from build123d import *

# Parameters (mm, degrees)
F0_R     = 2.5
F1_DEPTH = 7.5
F2_W     = 3.4
F2_H     = 15.4505071864
F2_W_2   = 3.8797123611
F2_W_3   = 3.8316924378
F3_DEPTH = 16.41578
F5_DEPTH = 2.8
F7_DEPTH = 2.8


with BuildPart() as f1:
    # F0 (on Right) → F1 (new body, symmetric)
    with BuildSketch(Plane.YZ):
        with BuildLine():
            Line((7.5, -12.5), (7.5, 0))
            ThreePointArc((7.5, 0), (0, 7.5), (-7.5, 0))
            Line((-7.5, 0), (-7.5, -12.5))
            Line((-7.5, -12.5), (7.5, -12.5))
        make_face()
        Circle(F0_R, mode=Mode.SUBTRACT)
    extrude(amount=F1_DEPTH, both=True)

    # F2 (on Front) → F3 (cut, symmetric)
    with BuildSketch(Plane.XZ):
        with Locations((0, 0.7252535932)):
            Rectangle(F2_W, F2_H)
        with Locations((-6.6398561805, 0.7252535932)):
            Rectangle(F2_W_2, F2_H)
        with Locations((6.6158462189, 0.7252535932)):
            Rectangle(F2_W_3, F2_H)
    extrude(amount=F3_DEPTH, both=True, mode=Mode.SUBTRACT)

    # F4 (on face) → F5 (cut, through all)
    with BuildSketch(Plane(origin=(-7.5, 0, 0), x_dir=(0, -1, 0), z_dir=(-1, 0, 0))):
        with BuildLine():
            ThreePointArc((2.6925824036, -7), (6.1824092402, -4.2459175671), (7.5, 0))
            ThreePointArc((7.5, 0), (-4.2459175671, 6.1824092402), (-2.6925824036, -7))
            Line((-2.6925824036, -7), (2.6925824036, -7))
        make_face()
        with BuildLine():
            Line((2.6925824036, -7), (-2.6925824036, -7))
            ThreePointArc((-2.6925824036, -7), (0, -7.5), (2.6925824036, -7))
        make_face()
    extrude(amount=-F5_DEPTH, mode=Mode.SUBTRACT)

    # F6 (on face) → F7 (cut, through all)
    with BuildSketch(Plane.YZ.offset(7.5)):
        with BuildLine():
            Line((2.6925824036, -7), (-2.6925824036, -7))
            ThreePointArc((-2.6925824036, -7), (0, -7.5), (2.6925824036, -7))
        make_face()
        with BuildLine():
            ThreePointArc((2.6925824036, -7), (6.1824092402, -4.2459175671), (7.5, 0))
            ThreePointArc((7.5, 0), (-4.2459175671, 6.1824092402), (-2.6925824036, -7))
            Line((-2.6925824036, -7), (2.6925824036, -7))
        make_face()
    extrude(amount=-F7_DEPTH, mode=Mode.SUBTRACT)


solid = f1.part
Verification items for the finished model (mm, model axes). A direction names the side the tool comes from. Give positions to 0.01 mm unless a question says otherwise; leave off trailing zeros. Loops run counter-clockwise (first coordinate to the right, second up) from the corner with the lowest first, then second, coordinate; pieces in that order, holes last.
1) Sectioned sample at A-A, the plane y = 0. Enter the section's corners in (x, z).
2) Sectioned sample at C-C, the plane x = 3. Enter the section's corners in (y, z), then the cut area to 3 significant figures.
3) Sectioned sample at D-D, the plane y = -6. Enter the section's corners in (x, z), then the cut area to 4 significant figures.
4) Draft check along Y on faces 6 (the flat face through (-6, 5, -7)), 7 (the cylindrical face through (3.18, -0.54, -2.44)), 8 (the cylindrical face through (3.22, 0.16, 7.5)), 9 (the cylindrical face through (-6.1, 0, -7.5)). Enter one of: pulls with the +Y half, pulls with the -Y half, needs draft (parallel to the pull), parting line crosses it, or undercut.
5) Thickness scan on line 1 along X through (y, z) = (4.25, -5.75); line 2 along Z through (x, y) = (3.8, 0); line 3 along Z through (x, y) = (-1.5, 4.5). Record the ranges inside material, lowest first.
6) Depth check by flat-ended pin: pin 1 Ø6.5 at (y, z) = (0, 0) entering from -X; pin 2 Ø0.8 at (x, y) = (-6.5, 5) entering from +Z; pin 3 Ø4.5 at (y, z) = (-1, -2) entering from +X. Enter the tip coordinate at first touch or a pass-through.
7) Set-up check for faces 1 (the flat face through (6, 5, -7)), 2 (the flat face through (0, 0, -7)), 3 (the flat face through (-6, -5, -7)), 4 (the cylindrical face through (-3.22, -0.54, -2.44)), 5 (the cylindrical face through (-3.18, 0.16, 7.5)): record each of +Z, -Z, +X, -X, +Y, -Y from which the full face is reachable in a straight line by a thin tool's end or side.
8) Sectioned sample at B-B, the plane z = -6.5. Enter the section's corners in (x, y), then the cut area to 3 significant figures.
Answers:
1. outline: (-7.5, -12.5) - (7.5, -12.5) - (7.5, -7.5) - (4.7, -7.5) - (4.7, -2.5) - (1.7, -2.5) - (1.7, -7) - (-1.7, -7) - (-1.7, -2.5) - (-4.7, -2.5) - (-4.7, -7.5) - (-7.5, -7.5) - close; (-4.7, 2.5) - (-1.7, 2.5) - (-1.7, 7.5) - (-4.7, 7.5) - close; (1.7, 2.5) - (4.7, 2.5) - (4.7, 7.5) - (1.7, 7.5) - close
2. outline: (-7.5, -12.5) - (7.5, -12.5) - (7.5, 0) arc R7.5 ccw to (-7.5, 0) - close; hole circle Ø5 at (0, 0)
2. area: 256 mm2
3. outline: (-7.5, -12.5) - (7.5, -12.5) - (7.5, -7) - (4.7, -7) - (4.7, 4.5) - (1.7, 4.5) - (1.7, -7) - (-1.7, -7) - (-1.7, 4.5) - (-4.7, 4.5) - (-4.7, -7) - (-7.5, -7) - close
3. area: 151.5 mm2
4. face 6: needs draft
4. face 7: undercut
4. face 8: parting line crosses it
4. face 9: undercut
5. line 1: x = -4.7 to -1.7, 1.7 to 4.7
5. line 2: z = -12.5 to -2.5, 2.5 to 7.5
5. line 3: z = -12.5 to -7
6. pin 1: stops at x = -4.7
6. pin 2: stops at z = -7
6. pin 3: stops at x = 4.7
7. face 1: +Z, +X, +Y, -Y
7. face 2: +Z, +Y, -Y
7. face 3: +Z, -X, +Y, -Y
7. face 4: +X, -X
7. face 5: +Z, +X, -X
8. outline: (-4.7, -7.5) - (-1.7, -7.5) - (-1.7, 7.5) - (-4.7, 7.5) - close; (1.7, -7.5) - (4.7, -7.5) - (4.7, 7.5) - (1.7, 7.5) - close
8. area: 90.0 mm2
